CAD build for the part. Positions are in the model's coordinates, mm. A direction names the side the tool comes from. Give positions to 0.01 mm unless a question says otherwise; leave off trailing zeros. Write each loop counter-clockwise with the first axis right and the second up, starting at its lowest first coordinate (ties: lowest second). Pieces come first, ordered by that corner, then holes. Notation, with made-up numbers: (16.5, 47.25) -> (57.5, 47.25) arc R26 ccw to (57.5, 80.25) -> close; hole circle Ø6 at (87.25, 38.5). An arc over 180 degrees is marked (long way). Answer as a JSON object with one key per item and string values.
Autodesk Inventor part; units mm, degrees
ref_plane "YZ Plane" through (0, 0, 0) normal (1, 0, 0) x (0, 1, 0)
ref_plane "XZ Plane" through (0, 0, 0) normal (0, 1, 0) x (-1, 0, 0)
ref_plane "XY Plane" through (0, 0, 0) normal (0, 0, 1) x (1, 0, 0)
sketch "Sketch1" plane through (0, 0, 0) normal (0, 0, 1) x (1, 0, 0)
  line L0 (0, 0) -> (0, 76.2)
  line L1 (0, 0) -> (50.8, 0)
  line L2 (50.8, 0) -> (50.8, -12.7)
  line L3 (50.8, -12.7) -> (114.3, -12.7)
  line L4 (114.3, -12.7) -> (114.3, -25.4)
  line L5 (0, 76.2) -> (-5.5192, 76.2)
  arc A0 (-5.5192, 76.2) -> (-17.9219, 66.232) centre (-5.5192, 63.5) ccw
  arc A1 (-31.0067, 6.83) -> (0, -31.75) centre (0, 0) ccw
  line L6 (-17.9219, 66.232) -> (-31.0067, 6.83)
  line L7 (0, -31.75) -> (19.05, -31.75)
  line L8 (6.35, -31.1085) -> (6.35, -31.75)
  line L9 (19.05, -31.75) -> (19.05, -44.45)
  line L10 (19.05, -44.45) -> (88.9, -44.45)
  line L11 (88.9, -44.45) -> (114.3, -25.4)
  dimension "d0" = 76.2
  dimension "d1" = 50.8
  dimension "d2" = 12.7
  dimension "d3" = 63.5
  dimension "d4" = 12.7
  dimension "d13" = 19.05
  dimension "d15" = 12.7
  dimension "d16" = 69.85
  dimension "d17" = 31.75
  dimension "d18" = 59.402
extrude "Extrusion1" add sketch "Sketch1" against normal blind 76.2
sketch "Sketch2" plane through (0, 0, 0) normal (0, 1, 0) x (1, 0, 0)
  line L0 (50.8, 0) -> (50.8, 76.2)
  circle A0 centre (50.8, 38.1) radius 38.1
  point P0 (0, 0)
extrude "Extrusion2" add sketch "Sketch2" against normal blind 12.7
sketch "Sketch3" plane through (0, 0, 0) normal (0, 1, 0) x (1, 0, 0)
  arc A0 (50.8, 0) -> (50.8, 76.2) centre (50.8, 38.1) ccw
  circle A1 centre (50.8, 38.1) radius 19.05
  point P0 (0, 0)
  dimension "d24" = 38.1
extrude "Extrusion3" cut sketch "Sketch3" against normal through all
properties part number "5.4"
1) Mould opens along Z. For faces 4 (the flat face through (25, -2, -76.2)), 5 (the cylindrical face through (-13.381, 73.474, -37.567)), 6 (the cylindrical face through (35.68, -21.91, -26.51)) say: released by +Z, released by -Z, zero draft, split by the parting line, or undercut.
Model answer:
{"face 4": "released by -Z", "face 5": "zero draft", "face 6": "undercut"}
2) Slice it at A-A (z = -38.1). List the corners of the cut face in (x, y).
Model answer:
{"outline": "(-31.01, 6.83) arc R31.75 ccw to (0, -31.75) -> (19.05, -31.75) -> (19.05, -44.45) -> (31.75, -44.45) -> (31.75, 0) -> (0, 0) -> (0, 76.2) -> (-5.52, 76.2) arc R12.7 ccw to (-17.92, 66.23) -> close; (69.85, -44.45) -> (88.9, -44.45) -> (114.3, -25.4) -> (114.3, -12.7) -> (88.9, -12.7) -> (88.9, 0) -> (69.85, 0) -> close"}
3) Slice it at D-D (x = 98.5). List the corners of the cut face in (y, z), then the cut area to 3 significant figures.
Model answer:
{"outline": "(-37.25, -76.2) -> (-12.7, -76.2) -> (-12.7, 0) -> (-37.25, 0) -> close", "area": "1,870 mm2"}
4) Pin check, flat tips, straight feed: pin 1 (2 mm diameter, centred on y = -8.5, z = -23, fed in from -X); pin 2 (5.5 mm diameter, centred on x = 10, z = -54.5, fed in from -Y); pin 3 (12 mm diameter, centred on x = 79, z = -46, fed in from +Y). Stop position of each tip, or through.
Model answer:
{"pin 1": "stops at x = -30.85", "pin 2": "stops at y = -31.75", "pin 3": "stops at y = 0"}
5) Slice it at B-B (y = -22). List the corners of the cut face in (x, z).
Model answer:
{"outline": "(-22.89, -76.2) -> (114.3, -76.2) -> (114.3, 0) -> (-22.89, 0) -> close; hole circle Ø38.1 at (50.8, -38.1)"}
6) Slice it at C-C (z = -16.5). List the corners of the cut face in (x, y), then the cut area to 3 significant figures.
Model answer:
{"outline": "(-31.01, 6.83) arc R31.75 ccw to (0, -31.75) -> (19.05, -31.75) -> (19.05, -44.45) -> (88.9, -44.45) -> (114.3, -25.4) -> (114.3, -12.7) -> (82.19, -12.7) -> (82.19, 0) -> (0, 0) -> (0, 76.2) -> (-5.52, 76.2) arc R12.7 ccw to (-17.92, 66.23) -> close", "area": "6,800 mm2"}
7) 3-axis set-ups, long thin cutter, end or side, ignore diameter. For faces 1 (the flat face through (9, -31.75, -38)), 2 (the cylindrical face through (88.89, -6.26, -37.26)), 3 (the flat face through (24, 0, -38)): which of +Z, -Z, +X, -X, +Y, -Y reach the whole face in a straight line?
Model answer:
{"face 1": "+Z, -Z, -X, -Y", "face 2": "+X, +Y", "face 3": "+Z, -Z, +X, +Y"}
8) Wall check: probe 1 along Z at (x, y) = (50, -18); probe 2 along Y at (x, z) = (58, -11.5); probe 3 along X at (y, z) = (-13.5, -38.1). Give the ranges that are in metal, low to high.
Model answer:
{"probe 1": "z = -76.2 to -57.13, -19.07 to 0", "probe 2": "y = -44.45 to 0", "probe 3": "x = -28.74 to 31.75, 69.85 to 114.3"}
